from build123d import *

# Parameters (mm, degrees)
SKETCH_1_W          = 30
SKETCH_1_H          = 20
SKETCH_1_W_2        = 26
SKETCH_1_H_2        = 16
EXTRUDE_1_DEPTH     = 560
SKETCH_3_R          = 2.5
CUT_EXTRUDE_2_DEPTH = 561.557757952
SKETCH_4_R          = 2.5
CUT_EXTRUDE_3_DEPTH = 561.557757952
SKETCH_7_R          = 3
CUT_EXTRUDE_5_DEPTH = 30
SKETCH_8_R          = 2.5
CUT_EXTRUDE_6_DEPTH = 30
SKETCH_10_R         = 2.5
CUT_EXTRUDE_7_DEPTH = 30
SKETCH_11_R         = 2.5
CUT_EXTRUDE_8_DEPTH = 30


with BuildPart() as part:
    # 草图1 → 凸台-拉伸1 (new body)
    with BuildSketch(Plane.XY):
        Rectangle(SKETCH_1_W, SKETCH_1_H)
        Rectangle(SKETCH_1_W_2, SKETCH_1_H_2, mode=Mode.SUBTRACT)
    extrude(amount=EXTRUDE_1_DEPTH)

    # 草图3 → 切除-拉伸2 (cut, through all)
    with BuildSketch(Plane(origin=(0, 10, 0), x_dir=(1, 0, 0), z_dir=(0, 1, 0))):
        with Locations(Location((-7.5, -10, 0), (0, 0, 180))):
            Circle(SKETCH_3_R)
        with Locations(Location((7.5, -10, 0), (0, 0, 180))):
            Circle(SKETCH_3_R)
    extrude(amount=-CUT_EXTRUDE_2_DEPTH, mode=Mode.SUBTRACT)

    # 草图4 → 切除-拉伸3 (cut, through all)
    with BuildSketch(Plane(origin=(0, 10, 0), x_dir=(1, 0, 0), z_dir=(0, 1, 0))):
        with Locations(Location((-7.5, -312.5, 0), (0, 0, 180))):
            Circle(SKETCH_4_R)
        with Locations(Location((7.5, -312.5, 0), (0, 0, 180))):
            Circle(SKETCH_4_R)
    extrude(amount=-CUT_EXTRUDE_3_DEPTH, mode=Mode.SUBTRACT)

    # 草图7 → 切除-拉伸5 (cut)
    with BuildSketch(Plane.ZY.offset(15)):
        with Locations(Location((260, 0, 0), (0, 0, 270))):
            Circle(SKETCH_7_R)
        with Locations(Location((280, 0, 0), (0, 0, 270))):
            Circle(SKETCH_7_R)
        with Locations(Location((240, 0, 0), (0, 0, 270))):
            Circle(SKETCH_7_R)
    extrude(amount=-CUT_EXTRUDE_5_DEPTH, mode=Mode.SUBTRACT)

    # 草图8 → 切除-拉伸6 (cut)
    with BuildSketch(Plane(origin=(0, 10, 0), x_dir=(1, 0, 0), z_dir=(0, 1, 0))):
        with Locations(Location((0, -370, 0), (0, 0, 270))):
            Circle(SKETCH_8_R)
        with Locations(Location((0, -450, 0), (0, 0, 270))):
            Circle(SKETCH_8_R)
        with Locations(Location((0, -410, 0), (0, 0, 270))):
            Circle(SKETCH_8_R)
        with Locations(Location((0, -340, 0), (0, 0, 270))):
            Circle(SKETCH_8_R)
    extrude(amount=-CUT_EXTRUDE_6_DEPTH, mode=Mode.SUBTRACT)

    # 草图10 → 切除-拉伸7 (cut)
    with BuildSketch(Plane(origin=(0, 10, 0), x_dir=(1, 0, 0), z_dir=(0, 1, 0))):
        with Locations(Location((-7, -173, 0), (0, 0, 270))):
            Circle(SKETCH_10_R)
        with Locations(Location((7, -173, 0), (0, 0, 270))):
            Circle(SKETCH_10_R)
    extrude(amount=-CUT_EXTRUDE_7_DEPTH, mode=Mode.SUBTRACT)

    # 草图11 → 切除-拉伸8 (cut)
    with BuildSketch(Plane(origin=(0, 10, 0), x_dir=(1, 0, 0), z_dir=(0, 1, 0))):
        with Locations(Location((0, -85, 0), (0, 0, 270))):
            Circle(SKETCH_11_R)
        with Locations(Location((0, -115, 0), (0, 0, 270))):
            Circle(SKETCH_11_R)
        with Locations(Location((0, -203, 0), (0, 0, 270))):
            Circle(SKETCH_11_R)
        with Locations(Location((0, -233, 0), (0, 0, 270))):
            Circle(SKETCH_11_R)
        with Locations(Location((0, -145, 0), (0, 0, 270))):
            Circle(SKETCH_11_R)
    extrude(amount=-CUT_EXTRUDE_8_DEPTH, mode=Mode.SUBTRACT)


solid = part.part
Input: part model. Units: mm. Frame: model coordinates. A direction names the side the tool comes from. Give positions to 0.01 mm unless a question says otherwise; leave off trailing zeros. Write each loop counter-clockwise with the first axis right and the second up, starting at its lowest first coordinate (ties: lowest second). Pieces come first, ordered by that corner, then holes. Notation, with made-up numbers: (65, 37.5) -> (103, 37.5) arc R24 cw to (103, 60.5) -> close; hole circle Ø3 at (-36.5, -9). An arc over 180 degrees is marked (long way). Use one line per item in the form item = value. Start each with the question number.
1) Section query A-A on z = 70. Return the cut outline in (x, y), then the cut area to 3 significant figures.
2) Set-up query: faces 1 (the flat face through (-13, 0, 276)), 2 (the flat face through (0, 10, 276)). Return all of +Z, -Z, +X, -X, +Y, -Y with unobstructed straight access to the full face (end or side cutting, diameter ignored); none if empty.
3) Ray query, probe 1 along X at (y, z) = (-8.45, 312.5); probe 2 along X at (y, z) = (-9.25, 173); probe 3 along X at (y, z) = (-8.55, 340). Return the intervals inside material, ascending. Write a range as from..to.
4) Pin query (flat end, axial travel): pin 1 (5.5 mm diameter, centred on y = 0, z = 240, fed in from +X). Return the tip coordinate at first contact, or that it passes through.
5) Draft query along X for faces 3 (the flat face through (0, -9, 560)), 4 (the flat face through (15, 0, 276)), 5 (the flat face through (0, 8, 276)). Return one class per face: pulls with the +X half, pulls with the -X half, needs draft (parallel to the pull), parting line crosses it, or undercut.
Outcome:
q1.outline = (-15, -10) -> (15, -10) -> (15, 10) -> (-15, 10) -> close; hole (-13, -8) -> (13, -8) -> (13, 8) -> (-13, 8) -> close
q1.area = 184 mm^2
q2.face_1 = +Z, -Z
q2.face_2 = +Z, -Z, +X, -X, +Y
q3.probe_1 = -15..-10, -5..5, 10..15
q3.probe_2 = -15..-9.5, -4.5..4.5, 9.5..15
q3.probe_3 = -15..-2.5, 2.5..15
q4.pin_1 = through
q5.face_3 = needs draft
q5.face_4 = pulls with the +X half
q5.face_5 = undercut
